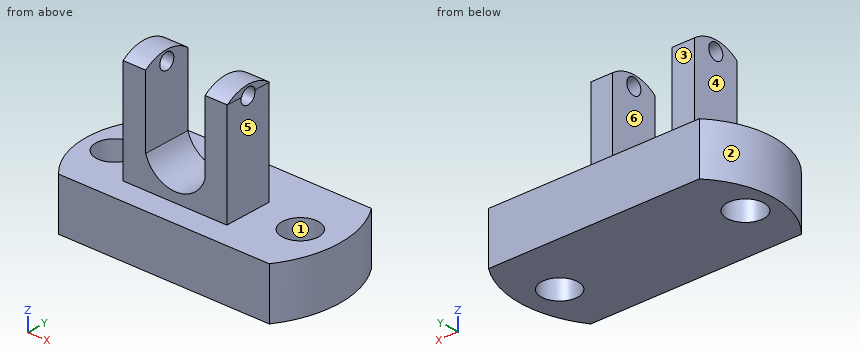
```python
from build123d import *

# Parameters (mm, degrees)
F0_W      = 52.1168857813
F0_H      = 28.5012163222
F1_DEPTH  = 12.7
F3_DEPTH  = 12.7
F5_DEPTH  = 12.7
F6_W      = 25.6421938539
F6_H      = 11.7544634268
F7_DEPTH  = 25.4
F9_DEPTH  = 25.781
F10_W     = 14.6912932396
F10_H     = 17.5639255852
F11_DEPTH = 22.5609156693
F12_R     = 4.5307401999
F12_R_2   = 4.4852627038
F13_DEPTH = 12.701
F14_R     = 1.9651697752
F15_DEPTH = 45.8603734278
F17_DEPTH = 22.5609156693


with BuildPart() as f1:
    # F0 (on Top) → F1 (new body)
    with BuildSketch(Plane.XY):
        with Locations((-10.29464975, 14.2506081611)):
            Rectangle(F0_W, F0_H)
    extrude(amount=F1_DEPTH)

    # F2 (on face) → F3 (join)
    with BuildSketch(Plane.XY.offset(12.7)):
        with BuildLine():
            Line((-36.3530926406, 0), (-36.3530926406, 28.5012163222))
            ThreePointArc((-36.3530926406, 28.5012163222), (-41.8927435543, 14.2506081611), (-36.3530926406, 0))
        make_face()
    extrude(amount=-F3_DEPTH)

    # F4 (on face) → F5 (join)
    with BuildSketch(Plane.XY.offset(12.7)):
        with BuildLine():
            Line((15.7637931406, 28.5012163222), (15.7637931406, 0))
            ThreePointArc((15.7637931406, 0), (20.217179574, 14.2506081611), (15.7637931406, 28.5012163222))
        make_face()
    extrude(amount=-F5_DEPTH)

    # F6 (on face) → F7 (join)
    with BuildSketch(Plane.XY.offset(12.7)):
        with Locations((-12.8210969269, 11.8185323663)):
            Rectangle(F6_W, F6_H)
    extrude(amount=F7_DEPTH)

    # F8 (on face) → F9 (join)
    with BuildSketch(Plane(origin=(-25.6421938539, 0, 0), x_dir=(0, -1, 0), z_dir=(-1, 0, 0))):
        with BuildLine():
            Line((-17.6957640797, 38.1), (-5.9413006529, 38.1))
            ThreePointArc((-5.9413006529, 38.1), (-11.8185323663, 40.0893589301), (-17.6957640797, 38.1))
        make_face()
    extrude(amount=-F9_DEPTH)

    # F10 (on face) → F11 (cut, through all)
    with BuildSketch(Plane.XZ.offset(-5.9413006529)):
        Polygon((-5.3697098047, 40.5042394996), (-20.0610030442, 40.2643792331), (-20.0610030442, 38.1), (-5.3697098047, 38.1), align=None)
        with Locations((-12.7153564245, 29.3180372074)):
            Rectangle(F10_W, F10_H)
    extrude(amount=-F11_DEPTH, mode=Mode.SUBTRACT)

    # F12 (on face) → F13 (cut, through all)
    with BuildSketch(Plane.XY.offset(12.7)):
        with Locations((-34.616753459, 13.6625757441)):
            Circle(F12_R)
        with Locations((11.228363961, 13.7757733464)):
            Circle(F12_R_2)
    extrude(amount=-F13_DEPTH, mode=Mode.SUBTRACT)

    # F14 (on face) → F15 (cut, through all)
    with BuildSketch(Plane(origin=(-25.6421938539, 0, 0), x_dir=(0, -1, 0), z_dir=(-1, 0, 0))):
        with Locations((-11.8185323663, 37.5899001956)):
            Circle(F14_R)
    extrude(amount=-F15_DEPTH, mode=Mode.SUBTRACT)

    # F16 (on face) → F17 (cut, through all)
    with BuildSketch(Plane.XZ.offset(-5.9413006529)):
        with BuildLine():
            Line((-5.3697098047, 20.5360744148), (-20.0610030442, 20.5360744148))
            ThreePointArc((-20.0610030442, 20.5360744148), (-12.7153564245, 15.1077599737), (-5.3697098047, 20.5360744148))
        make_face()
    extrude(amount=-F17_DEPTH, mode=Mode.SUBTRACT)


solid = f1.part
```
For this review, take the finished solid that the model builds, in its own axes (mm). Face numbers are marked on the shaded views. A direction names the side the tool comes from. Coordinates: 2 decimals unless noted, no trailing zeros. Write each loop counter-clockwise with the first axis right and the second up, starting at its lowest first coordinate (ties: lowest second). Pieces come first, ordered by that corner, then holes. Notation, with made-up numbers: (56.5, 26) - (72.5, 26) arc R23 ccw to (72.5, 59) - close; hole circle Ø11 at (-10.75, 78). An arc over 180 degrees is marked (long way). Answer in a Markdown table with one row per item. Add a question column.
Q1. Tool access review of the marked faces 4, 5 and 6: name each direction out of +Z, -Z, +X, -X, +Y, -Y from which nothing blocks a thin tool from reaching the whole face with its end or side.
Q2. We need section D-D, the plane x = -11.5. State the section outline as (y, z) points.
Q3. We need section B-B, the plane y = 15.25. State the section outline as (x, z) points.
Q4. We need section A-A, the plane z = 25. State the section outline as (x, y) points.
Q5. Draft analysis for pull direction X (two halves, no side actions). For the marked faces 1, 2 and 3, state which applies: +X half, -X half, draft (parallel to the pull), parting line (faces both ways), or undercut.
Q6. We need section C-C, the plane x = 9. State the section outline as (y, z) points.
Q7. For probe 1 along X at (y, z) = (13.75, 32); probe 2 along X at (y, z) = (11.5, 7.5); probe 3 along Z at (x, y) = (-6, 25.75), list the stretches that pass through material, from the lowest coordinate up.
Q8. For P1, Ø13, axis at y = 13.5, z = 23, coming from the -X side; P2, Ø1, axis at x = 2, z = 25, coming from the +Y side; P3, Ø8, axis at y = 18.5, z = 7.5, coming from the +X side; P4, Ø13, axis at y = 10.5, z = 31.5, coming from the +X side, all flat-tipped, find the tip position at first contact; note any pin that passes through.
Answer list:
| question | item | result |
|---|---|---|
| 1 | face 4 | +Z, -X, +Y, -Y |
| 1 | face 5 | +X, +Y, -Y |
| 1 | face 6 | +Z, +Y, -Y |
| 2 | outline | (0, 0) - (28.5, 0) - (28.5, 12.7) - (17.7, 12.7) - (17.7, 15.2) - (5.94, 15.2) - (5.94, 12.7) - (0, 12.7) - close |
| 3 | outline | (-41.87, 0) - (-38.86, 0) - (-38.86, 12.7) - (-41.87, 12.7) - close; (-30.37, 0) - (6.99, 0) - (6.99, 12.7) - (0, 12.7) - (0, 38.1) - (0.14, 38.1) - (0.14, 39.46) - (-5.37, 39.46) - (-5.37, 20.54) arc R7.68 cw to (-20.06, 20.54) - (-20.06, 39.46) - (-25.64, 39.46) - (-25.64, 12.7) - (-30.37, 12.7) - close; (15.46, 0) - (20.2, 0) - (20.2, 12.7) - (15.46, 12.7) - close |
| 4 | outline | (-25.64, 5.94) - (-20.06, 5.94) - (-20.06, 17.7) - (-25.64, 17.7) - close; (-5.37, 5.94) - (0, 5.94) - (0, 17.7) - (-5.37, 17.7) - close |
| 5 | face 1 | undercut |
| 5 | face 2 | -X half |
| 5 | face 3 | draft |
| 6 | outline | (0, 0) - (9.88, 0) - (9.88, 12.7) - (0, 12.7) - close; (17.67, 0) - (28.5, 0) - (28.5, 12.7) - (17.67, 12.7) - close |
| 7 | probe 1 | x = -25.64 to -20.06, -5.37 to 0 |
| 7 | probe 2 | x = -41.71 to -38.6, -30.64 to 7.36, 15.09 to 20.07 |
| 7 | probe 3 | z = 0 to 12.7 |
| 8 | P1 | stops at x = -25.64 |
| 8 | P2 | passes through |
| 8 | P3 | stops at x = 20.22 |
| 8 | P4 | stops at x = 0 |
